Geometry check sheet. Reference: the model listing, model coordinates, mm. Face numbers are marked on the shaded views. Coordinates: 2 decimals unless noted, no trailing zeros. Loops run counter-clockwise (first coordinate to the right, second up) from the corner with the lowest first, then second, coordinate; pieces in that order, holes last.
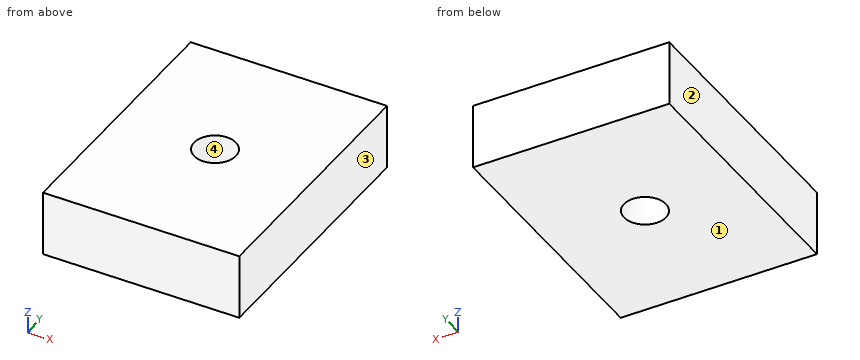
from build123d import *

# Parameters (mm, degrees)
F1_DEPTH = 5


with BuildPart() as f1:
    # F0 (on Top) → F1 (new body)
    with BuildSketch(Plane.XY):
        with BuildLine():
            Line((0, 10), (0, 0))
            Line((0, 0), (15, 0))
            Line((15, 0), (15, 10))
            Line((15, 10), (9.1, 10))
            ThreePointArc((9.1, 10), (7.5, 8.4), (5.9, 10))
            Line((5.9, 10), (0, 10))
        make_face()
        with BuildLine():
            Line((0, 20), (0, 10))
            Line((0, 10), (5.9, 10))
            ThreePointArc((5.9, 10), (7.5, 11.6), (9.1, 10))
            Line((9.1, 10), (15, 10))
            Line((15, 10), (15, 20))
            Line((15, 20), (0, 20))
        make_face()
    extrude(amount=F1_DEPTH)


solid = f1.part
(1) Sectioned sample at B-B on y = 10. Record the cut outline in (x, z).
Findings:
outline: (0, 0) - (5.9, 0) - (5.9, 5) - (0, 5) - close; (9.1, 0) - (15, 0) - (15, 5) - (9.1, 5) - close
(2) Draft check along X on the marked faces 1, 2, 3 and 4. Enter one of: +X half, -X half, draft (parallel to the pull), parting line (faces both ways), or undercut.
Findings:
face 1: draft
face 2: -X half
face 3: +X half
face 4: undercut
(3) Sectioned sample at A-A on x = 7.5. Record the cut outline in (y, z).
Findings:
outline: (0, 0) - (8.4, 0) - (8.4, 5) - (0, 5) - close; (11.6, 0) - (20, 0) - (20, 5) - (11.6, 5) - close
(4) Sectioned sample at C-C on z = 1.7. Record the cut outline in (x, y).
Findings:
outline: (0, 0) - (15, 0) - (15, 20) - (0, 20) - close; hole circle Ø3.2 at (7.5, 10)
(5) Scan lines: L1, parallel to Y at x = 7.5, z = 3.1; L2, parallel to X at y = 10.5, z = 4.05; L3, parallel to Y at x = 7, z = 3.45. Record each from-to range of solid material in increasing order.
Findings:
L1: y = 0 to 8.4, 11.6 to 20
L2: x = 0 to 5.98, 9.02 to 15
L3: y = 0 to 8.48, 11.52 to 20
(6) Gauge pin test, flat end, axial feed: pin 1 Ø3.5 at (x, y) = (7.5, 10) entering from -Z. Record the tip position at first contact, or that the pin passes through.
Findings:
pin 1: stops at z = 0
